Could you check a few things on this model? Use its own coordinates, in mm. Give positions to 0.01 mm unless a question says otherwise; leave off trailing zeros. Loops run counter-clockwise (first coordinate to the right, second up) from the corner with the lowest first, then second, coordinate; pieces in that order, holes last. Notation, with made-up numbers: M 83,-7.75 L 118,-7.75 A10 ccw 118,-1.75 Z; hole C 69,-31.75 d9. An arc over 180 degrees is marked long. Answer in a Markdown table with one row per item. Add a question column.
1. If we section it at A-A on y = -162.5: List the corners of the cut face in (x, z) for me, then the cut area to 3 significant figures.
2. I'm going to push flat-ended pins straight in: pin 1 Ø5 at (y, z) = (57, 138.5) entering from -X; pin 2 Ø5 at (x, y) = (473.5, 225) entering from +Z; pin 3 Ø3 at (y, z) = (-136, 57) entering from +X. Where does each tip first touch, or does it pass through?
3. Thinking about a two-plate mould opening in Y: for faces 1 (the cylindrical face through (304.418, 336.098, 285.175)), 2 (the flat face through (251.68, 321.02, 371.84)), 3 (the flat face through (250.44, -320.34, 373.88)), which applies, released by +Y, released by -Y, zero draft, split by the parting line, or undercut?
4. I need wall thicknesses on line 1 along Z through (x, y) = (400, -233); line 2 along X through (y, z) = (-262.5, 170); line 3 along X through (y, z) = (-305.5, 270). Which ranges of each line are inside material? Lowest first, please. Write a range as from..to.
5. If we section it at B-B on z = -5.5: List the corners of the cut face in (x, y) for me, then the cut area to 3 significant figures.
```python
from build123d import *

# Parameters (mm, degrees)
BOSS_EXTRUDE1_DEPTH = 0.3175
SKETCH4_R           = 12.8905
CUT_EXTRUDE1_DEPTH  = 152.4
SKETCH5_R           = 12.8905
CUT_EXTRUDE2_DEPTH  = 152.4
SKETCH6_R           = 12.8905
CUT_EXTRUDE3_DEPTH  = 152.4


with BuildPart() as part:
    # Sketch3 → Boss-Extrude1 (new body, symmetric)
    with BuildSketch(Plane(origin=(348.778890993, 0, 212.329779666), x_dir=(0.519999813, 0, -0.854166374), z_dir=(0.854166374, 0, 0.519999813))):
        Polygon((310.98364901, 0), (310.98364901, 336.55), (-63.66635099, 356.184574508), (-273.21635099, 296.314909512), (-273.21635099, 0), align=None)
        Polygon((310.98364901, -336.55), (310.98364901, 0), (-273.21635099, 0), (-273.21635099, -296.314909512), (-63.66635099, -356.184574508), align=None)
    extrude(amount=BOSS_EXTRUDE1_DEPTH, both=True)

    # Sketch4 → Cut-Extrude1 (cut)
    with BuildSketch(Plane(origin=(381.685291714, 370.332, -52.606299668), x_dir=(0, 0, 1), z_dir=(-0.956162433, 0.292836818, 0))):
        Circle(SKETCH4_R)
    cut_extrude1 = extrude(amount=-CUT_EXTRUDE1_DEPTH, mode=Mode.SUBTRACT)

    # Sketch5 → Cut-Extrude2 (cut)
    with BuildSketch(Plane(origin=(197.535291714, 368.359946538, 264.893700332), x_dir=(0.030514213, -0.004769179, 0.999522955), z_dir=(-0.987534126, 0.154345353, 0.030884661))):
        Circle(SKETCH5_R)
    cut_extrude2 = extrude(amount=-CUT_EXTRUDE2_DEPTH, mode=Mode.SUBTRACT)

    # Sketch6 → Cut-Extrude3 (cut)
    with BuildSketch(Plane(origin=(197.535291714, 368.359946538, 264.893700332), x_dir=(-0.218520162, 0.041163819, 0.974963835), z_dir=(-0.958112576, 0.180484822, -0.222363489))):
        Circle(SKETCH6_R)
    cut_extrude3 = extrude(amount=-CUT_EXTRUDE3_DEPTH, mode=Mode.SUBTRACT)

    # Mirror1: Cut-Extrude1, Cut-Extrude2, Cut-Extrude3 across plane
    add(cut_extrude1.mirror(Plane.ZX), mode=Mode.SUBTRACT)
    add(cut_extrude2.mirror(Plane.ZX), mode=Mode.SUBTRACT)
    add(cut_extrude3.mirror(Plane.ZX), mode=Mode.SUBTRACT)


solid = part.part
```
Results:
| question | item | result |
|---|---|---|
| 1 | outline | M 206.44,445.54 L 510.22,-53.47 L 510.76,-53.14 L 206.98,445.87 Z |
| 1 | area | 371 mm2 |
| 2 | pin 1 | x = 391.83 |
| 2 | pin 2 | z = 12.18 |
| 2 | pin 3 | x = 444.63 |
| 3 | face 1 | undercut |
| 3 | face 2 | released by +Y |
| 3 | face 3 | released by -Y |
| 4 | line 1 | 127.58..128.8 |
| 4 | line 2 | 374.18..374.92 |
| 4 | line 3 | 313.3..314.04 |
| 5 | outline | M 481.02,-339.49 L 481.76,-339.47 L 481.76,339.47 L 481.02,339.49 Z |
| 5 | area | 505 mm2 |
